```python
from build123d import *

# Parameters (mm, degrees)
SKETCH_1_W             = 46.5
SKETCH_1_H             = 20
EXTRUDE_1_DEPTH        = 3
EXTRUDE_2_DEPTH        = 3
PATTERN_LINEAR_1_COUNT = 14
PATTERN_LINEAR_1_PITCH = 3.141592654
SKETCH_3_R             = 1.65
CUT_EXTRUDE_1_DEPTH    = 3
SKETCH_4_R             = 1.65
SKETCH_4_R_2           = 1.5
CUT_EXTRUDE_2_DEPTH    = 10
CHAMFER_1_SIZE         = 5


with BuildPart() as part:
    # 草圖1 → 填料-伸長1 (new body)
    with BuildSketch(Plane.XY):
        Rectangle(SKETCH_1_W, SKETCH_1_H)
    extrude(amount=EXTRUDE_1_DEPTH)

    # 草圖2 → 填料-伸長2 (add)
    with BuildSketch(Plane.XY.offset(3)):
        Polygon((-22.25, 10), (-21.431066973, 12.25), (-20.588211115, 12.25), (-19.769278088, 10), align=None)
    extrude_2 = extrude(amount=-EXTRUDE_2_DEPTH)

    # 直線複製排列1: 填料-伸長2 ×14
    with Locations(*[(i * PATTERN_LINEAR_1_PITCH, 0, 0) for i in range(1, PATTERN_LINEAR_1_COUNT)]):
        add(extrude_2)

    # 草圖3 → 除料-伸長1 (cut)
    with BuildSketch(Plane.XY.offset(3)):
        with Locations((-10.25, 6)):
            Circle(SKETCH_3_R)
        with Locations((-2.25, 6)):
            Circle(SKETCH_3_R)
        with Locations((-2.25, -6)):
            Circle(SKETCH_3_R)
        with Locations((-10.25, -6)):
            Circle(SKETCH_3_R)
    extrude(amount=-CUT_EXTRUDE_1_DEPTH, mode=Mode.SUBTRACT)

    # 草圖4 → 除料-伸長2 (cut)
    with BuildSketch(Plane.XY.offset(3)):
        with Locations((15.05, 5)):
            Circle(SKETCH_4_R)
        with Locations((15.05, -5)):
            Circle(SKETCH_4_R_2)
    extrude(amount=-CUT_EXTRUDE_2_DEPTH, mode=Mode.SUBTRACT)

    # 導角1
    chamfer_1_edges = [part.edges().sort_by_distance(p)[0] for p in [
        (23.25, -10, 1.5),
        (-23.25, -10, 1.5),
    ]]
    chamfer(chamfer_1_edges, length=CHAMFER_1_SIZE)


solid = part.part
```
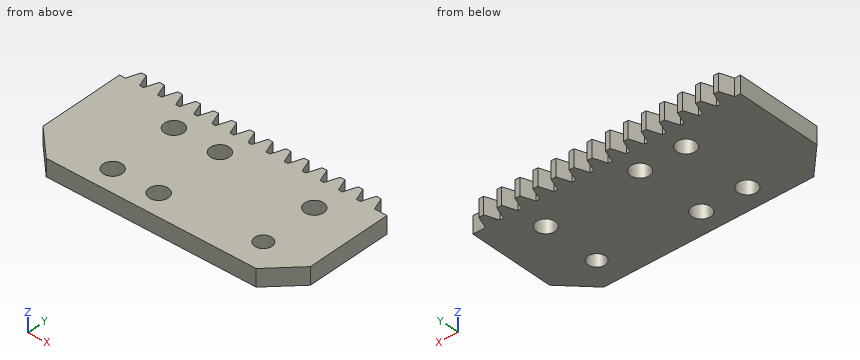
For this review, take the finished solid that the model builds, in its own axes (mm). Give positions to 0.01 mm unless a question says otherwise; leave off trailing zeros. Write each loop counter-clockwise with the first axis right and the second up, starting at its lowest first coordinate (ties: lowest second). Pieces come first, ordered by that corner, then holes. Notation, with made-up numbers: M -33.75,85 L 16.25,85 A21 ccw 16.25,98 Z; hole C 68,22.5 d7. An arc over 180 degrees is marked long. Answer as a JSON object with one key per item and string values. Group by question number.
Item 1: For probe 1 along Y at (x, z) = (15, 1.45); probe 2 along Y at (x, z) = (-2.25, 1.6); probe 3 along X at (y, z) = (-7.25, 2.75), list the stretches that pass through material, from the lowest coordinate up. Write a range as [from, to].
Item 2: Consider section C-C on y = -8.5. Write out the cut boundary in (x, z), plus the area to 4 significant figures.
Item 3: Consider section B-B on z = 1.7. Count the separate pieces of the cut face and the enclosed holes in it, plus the area to 3 significant figures.
Item 4: Consider section D-D on y = 6. Write out the cut boundary in (x, z), plus the area to 3 significant figures.
Item 5: Consider section A-A on y = -6. Write out the cut boundary in (x, z).
Check result:
{
 "1": {"probe 1": "y = [-10, -6.5], [-3.5, 3.35], [6.65, 10]", "probe 2": "y = [-10, -7.65], [-4.35, 4.35], [7.65, 12.25]", "probe 3": "x = [-21, -11.33], [-9.17, -3.33], [-1.17, 21]"},
 "2": {"outline": "M -19.75,0 L 19.75,0 L 19.75,3 L -19.75,3 Z", "area": "118.5 mm^2"},
 "3": {"separate pieces": "1", "enclosed holes": "6", "area": "908 mm^2"},
 "4": {"outline": "M -23.25,0 L -11.9,0 L -11.9,3 L -23.25,3 Z; M -8.6,0 L -3.9,0 L -3.9,3 L -8.6,3 Z; M -0.6,0 L 13.74,0 L 13.74,3 L -0.6,3 Z; M 16.36,0 L 23.25,0 L 23.25,3 L 16.36,3 Z", "area": "112 mm^2"},
 "5": {"outline": "M -22.25,0 L -11.9,0 L -11.9,3 L -22.25,3 Z; M -8.6,0 L -3.9,0 L -3.9,3 L -8.6,3 Z; M -0.6,0 L 13.93,0 L 13.93,3 L -0.6,3 Z; M 16.17,0 L 22.25,0 L 22.25,3 L 16.17,3 Z"}
}
